Read the model definition and answer for the solid it produces. Units are mm, in the model's axes. Face numbers are marked on the shaded views. A direction names the side the tool comes from. Round coordinates to 2 decimals unless told otherwise and drop trailing zeros. Order: outer loops, then holes, each group sorted by start corner. A loop starts at its lowest first (then second) coordinate and runs counter-clockwise, first axis right, second up. Notation, with made-up numbers: M 70.25,-28 L 98.25,-28 A30 cw 98.25,-3 Z; hole C 59,42 d3. An arc over 180 degrees is marked long. Answer as CSV lines item,"result".
Autodesk Inventor part; units mm, degrees
ref_plane "YZ Plane" through (0, 0, 0) normal (1, 0, 0) x (0, 1, 0)
ref_plane "XZ Plane" through (0, 0, 0) normal (0, 1, 0) x (-1, 0, 0)
ref_plane "XY Plane" through (0, 0, 0) normal (0, 0, 1) x (1, 0, 0)
sketch "Sketch1" plane through (0, 0, 0) normal (0, 1, 0) x (-1, 0, 0)
  circle A0 centre (0, 0) radius 40
  point P0 (20, 0)
  point P1 (14.1421, 14.1421)
  point P2 (0, 20)
  point P3 (-14.1421, 14.1421)
  point P4 (-20, 0)
  point P5 (-14.1421, -14.1421)
  point P6 (0, -20)
  point P7 (14.1421, -14.1421)
  point P8 (30, 0)
  point P9 (21.2132, 21.2132)
  point P10 (0, 30)
  point P11 (-21.2132, 21.2132)
  point P12 (-30, 0)
  point P13 (-21.2132, -21.2132)
  point P14 (0, -30)
  point P15 (21.2132, -21.2132)
  dimension "d0" = 80
  dimension "d2" = 20
  dimension "d5" = 360
  dimension "d31" = 30
  dimension "d34" = 360
extrude "Extrusion1" add sketch "Sketch1" against normal blind 15
hole "Hole1" at (-14.1421, 0, 14.1421) at (-14.1421, 0, -14.1421) at (14.1421, 0, 14.1421) at (14.1421, 0, -14.1421) direction (0, -1, 0) diameter 6.6 end through all counterbore diameter 11 counterbore depth 8
sketch "Sketch2" plane through (0, -15, 0) normal (0, -1, 0) x (1, 0, 0)
  circle A0 centre (0, 0) radius 40
  circle A1 centre (0, 20) radius 3
  circle A2 centre (0, -20) radius 3
  point P0 (20, 0)
  point P1 (14.1421, 14.1421)
  point P2 (-14.1421, 14.1421)
  point P3 (-20, 0)
  point P4 (-14.1421, -14.1421)
  point P5 (14.1421, -14.1421)
  dimension "d18" = 80
  dimension "d19" = 20
  dimension "d20" = 360
  dimension "d21" = 6
  dimension "d22" = 6
extrude "Extrusion2" add sketch "Sketch2" along normal blind 3 contours A1 | A2
chamfer "Chamfer1" distance 1 angle 45 1 edges at (-3, -18, -20)
chamfer "Chamfer2" distance 1 angle 45 1 edges at (-3, -18, 20)
hole "Hole2" at (-30, 0, 0) at (-21.2132, 0, 21.2132) at (0, 0, 30) at (21.2132, 0, 21.2132) at (30, 0, 0) at (21.2132, 0, -21.2132) at (0, 0, -30) at (-21.2132, 0, -21.2132) direction (0, -1, 0) diameter 4.134 end through all
properties part number "plate_for_CFS055CA501U"
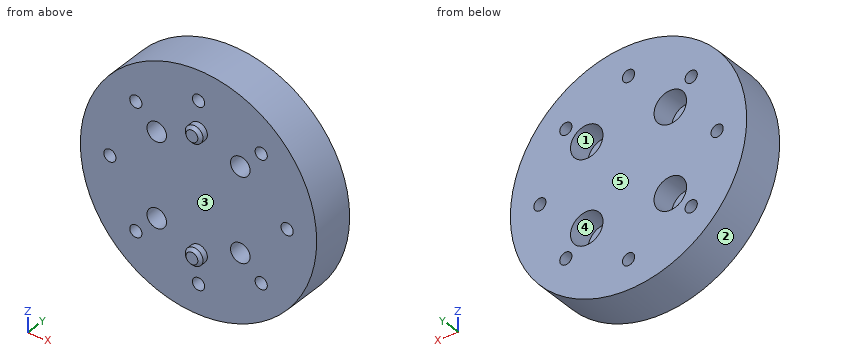
Item 1: Determine the mould class of the marked faces 1, 2 and 3 for opening direction X: +X half, -X half, draft (parallel to the pull), parting line (faces both ways), or undercut.
Ans:
face 1,"undercut"
face 2,"parting line"
face 3,"draft"
Item 2: A cutting plane is placed at A-A, the plane z = 0. Determine the outline of the cut face in (x, y).
Ans:
outline,"M -40,-15 L -32.07,-15 L -32.07,0 L -40,0 Z; M -27.93,-15 L 27.93,-15 L 27.93,0 L -27.93,0 Z; M 32.07,-15 L 40,-15 L 40,0 L 32.07,0 Z"
Item 3: A cutting plane is placed at D-D, the plane y = -6.5. Give the number of separate pieces and of enclosed holes in the cut face, and give its area (3 significant figures).
Ans:
separate pieces,"1"
enclosed holes,"12"
area,"4,540 mm2"
Item 4: A cutting plane is placed at C-C, the plane y = -16. Determine the outline of the cut face in (x, z).
Ans:
outline,"C 0,-20 d6; C 0,20 d6"
Item 5: A cutting plane is placed at B-B, the plane x = -30. Determine the outline of the cut face in (y, z), and give its area (3 significant figures).
Ans:
outline,"M -15,-26.46 L 0,-26.46 L 0,-2.07 L -15,-2.07 Z; M -15,2.07 L 0,2.07 L 0,26.46 L -15,26.46 Z"
area,"732 mm2"
Item 6: A tool of negligible diameter and unlimited length cuts with its end or side. For the marked faces 4 and 5, from which of +Z, -Z, +X, -X, +Y, -Y can it reach the whole face along a straight path? Write none if from no direction.
Ans:
face 4,"+Y"
face 5,"+Z, -Z, +X, -X, +Y"
Item 7: Flat-ended cylindrical pins translate along their axes: pin 1 (5.5 mm diameter, centred on x = 21.21, z = -21.21, fed in from -Y); pin 2 (10 mm diameter, centred on x = 14.14, z = -14.14, fed in from +Y); pin 3 (3.5 mm diameter, centred on x = 0, z = 30, fed in from +Y); pin 4 (1.5 mm diameter, centred on x = -30, y = -7.5, fed in from +Z). Find the tip coordinate at first contact, or state that the pin passes through.
Ans:
pin 1,"y = -15"
pin 2,"y = -8"
pin 3,"through"
pin 4,"z = 27.28"
Item 8: Find the intervals of material crossed by probe 1 along Z at (x, y) = (12, -12); probe 2 along Z at (x, y) = (16, -9); probe 3 along X at (y, z) = (-2.25, 11), in increasing order. Write a range as [from, to].
Ans:
probe 1,"[-38.16, -16.65], [-11.63, 11.63], [16.65, 38.16]"
probe 2,"[-36.66, -16.87], [-11.41, 11.41], [16.87, 36.66]"
probe 3,"[-38.46, -18.66], [-9.63, 9.63], [18.66, 38.46]"
